from build123d import *

# Parameters (mm, degrees)
BOSS_EXTRUDE1_DEPTH = 6
SKETCH2_W           = 6
SKETCH2_H           = 40
CUT_EXTRUDE1_DEPTH  = 10


with BuildPart() as part:
    # Sketch1 → Boss-Extrude1 (new body)
    with BuildSketch(Plane.XY):
        Polygon((-79, -40), (380, -40), (380, 40), (350.28, 40), (350.28, 14), (338.24, 14), (338.24, 40), (258.24, 40), (258.24, 14), (246.2, 14), (246.2, 40), (196.2, 40), (196.2, 14), (184.16, 14), (184.16, 40), (14.16, 40), (14.16, 14), (2.12, 14), (2.12, 40), (-79, 40), align=None)
    extrude(amount=BOSS_EXTRUDE1_DEPTH)

    # Sketch2 → Cut-Extrude1 (cut)
    with BuildSketch(Plane(origin=(0, 0, 0), x_dir=(-1, 0, 0), z_dir=(0, 0, -1))):
        with Locations((-67, 20)):
            Rectangle(SKETCH2_W, SKETCH2_H)
        with Locations((57, 20)):
            Rectangle(SKETCH2_W, SKETCH2_H)
        with Locations((-139, 20)):
            Rectangle(SKETCH2_W, SKETCH2_H)
    extrude(amount=-CUT_EXTRUDE1_DEPTH, mode=Mode.SUBTRACT)


solid = part.part
CAD build for the part. Positions are in the model's coordinates, mm. Round coordinates to 2 decimals unless told otherwise and drop trailing zeros. Order: outer loops, then holes, each group sorted by start corner. A loop starts at its lowest first (then second) coordinate and runs counter-clockwise, first axis right, second up. Notation, with made-up numbers: (69.25, -8) -> (109.25, -8) arc R29 ccw to (109.25, 28) -> close; hole circle Ø9 at (26, -0.5). An arc over 180 degrees is marked (long way). Write item = value, one per line. Start each with the question number.
(1) Cut at C-C, the plane y = 9. List the corners of the cut face in (x, z), then the cut area to 3 significant figures.
(2) Pin check, flat tips, straight feed: P1, Ø3, axis at x = 341.5, z = 3, coming from the +Y side; P2, Ø1.8, axis at x = -58, z = 2, coming from the +Y side. Stop position of each tip, or through.
(3) Cut at A-A, the plane y = 26.5. State how many separate pieces and enclosed holes the cut face has, then the cut area to 3 significant figures.
(4) Probe line 1 (X direction, y = 0.5, z = 3.95); line 2 (Y direction, x = 65, z = 1.2); line 3 (Y direction, x = 350, z = 5.55). List the from-to ranges inside material, lowest first. Write a range as [from, to].
Model answer:
q1.outline = (-79, 0) -> (-60, 0) -> (-60, 6) -> (-79, 6) -> close; (-54, 0) -> (64, 0) -> (64, 6) -> (-54, 6) -> close; (70, 0) -> (136, 0) -> (136, 6) -> (70, 6) -> close; (142, 0) -> (380, 0) -> (380, 6) -> (142, 6) -> close
q1.area = 2,650 mm2
q2.P1 = 14
q2.P2 = 0
q3.separate_pieces = 8
q3.enclosed_holes = 0
q3.area = 2,360 mm2
q4.line_1 = [-79, -60], [-54, 64], [70, 136], [142, 380]
q4.line_2 = [-40, 0]
q4.line_3 = [-40, 14]
